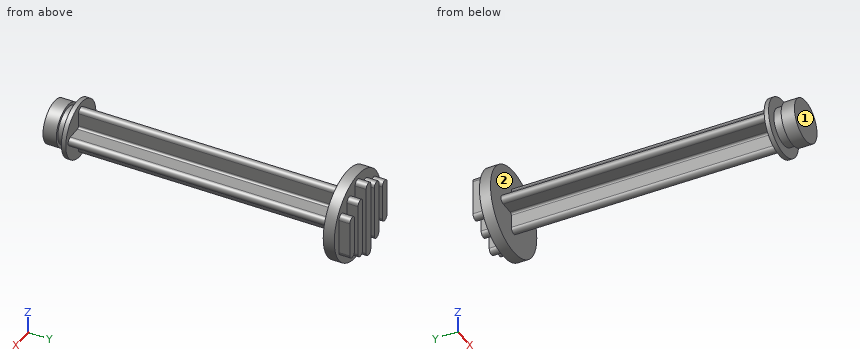
```python
from build123d import *

# Parameters (mm, degrees)
BOSS_EXTRUDE1_DEPTH = 60
SKETCH3_R           = 10
BOSS_EXTRUDE2_DEPTH = 2.5
BOSS_EXTRUDE3_DEPTH = 2.5


with BuildPart() as part:
    # Sketch1 → Revolve1 (revolve)
    with BuildSketch(Plane.XY):
        Polygon((0, 0), (4.875, 0), (4.875, 3), (4.225, 3), (4.225, 5), (6.5, 5), (6.5, 6), (0, 6), align=None)
    revolve(axis=Axis((0, 6, 0), (0, -1, 0)))

    # Sketch2 → Boss-Extrude1 (add)
    with BuildSketch(Plane(origin=(0, 6, 0), x_dir=(1, 0, 0), z_dir=(0, 1, 0))):
        with BuildLine():
            Line((-1, 4.5), (-1, 1.5))
            ThreePointArc((-1, 1.5), (-1.146446609, 1.146446609), (-1.5, 1))
            Line((-1.5, 1), (-4.5, 1))
            ThreePointArc((-4.5, 1), (-5.5, 0), (-4.5, -1))
            Line((-4.5, -1), (-1.5, -1))
            ThreePointArc((-1.5, -1), (-1.146446609, -1.146446609), (-1, -1.5))
            Line((-1, -1.5), (-1, -4.5))
            ThreePointArc((-1, -4.5), (0, -5.5), (1, -4.5))
            Line((1, -4.5), (1, -1.5))
            ThreePointArc((1, -1.5), (1.146446609, -1.146446609), (1.5, -1))
            Line((1.5, -1), (4.5, -1))
            ThreePointArc((4.5, -1), (5.5, 0), (4.5, 1))
            Line((4.5, 1), (1.5, 1))
            ThreePointArc((1.5, 1), (1.146446609, 1.146446609), (1, 1.5))
            Line((1, 1.5), (1, 4.5))
            ThreePointArc((1, 4.5), (0, 5.5), (-1, 4.5))
        make_face()
    extrude(amount=BOSS_EXTRUDE1_DEPTH)

    # Sketch3 → Boss-Extrude2 (add)
    with BuildSketch(Plane(origin=(0, 66, 0), x_dir=(1, 0, 0), z_dir=(0, 1, 0))):
        Circle(SKETCH3_R)
    extrude(amount=BOSS_EXTRUDE2_DEPTH)

    # Sketch4 → Boss-Extrude3 (add)
    with BuildSketch(Plane(origin=(0, 68.5, 0), x_dir=(1, 0, 0), z_dir=(0, 1, 0))):
        with BuildLine():
            ThreePointArc((1, 8), (0, 9), (-1, 8))
            Line((-1, 8), (-1, -8))
            ThreePointArc((-1, -8), (0, -9), (1, -8))
            Line((1, -8), (1, 8))
        make_face()
        with BuildLine():
            ThreePointArc((-2.5, 6), (-3.5, 7), (-4.5, 6))
            Line((-4.5, 6), (-4.5, -6))
            ThreePointArc((-4.5, -6), (-3.5, -7), (-2.5, -6))
            Line((-2.5, -6), (-2.5, 6))
        make_face()
        with BuildLine():
            ThreePointArc((4.5, 6), (3.5, 7), (2.5, 6))
            Line((2.5, 6), (2.5, -6))
            ThreePointArc((2.5, -6), (3.5, -7), (4.5, -6))
            Line((4.5, -6), (4.5, 6))
        make_face()
        with BuildLine():
            ThreePointArc((6, 4), (7, 5), (8, 4))
            Line((8, 4), (8, -4))
            ThreePointArc((8, -4), (7, -5), (6, -4))
            Line((6, -4), (6, 4))
        make_face()
        with BuildLine():
            Line((-6, -4), (-6, 4))
            ThreePointArc((-6, 4), (-7, 5), (-8, 4))
            Line((-8, 4), (-8, -4))
            ThreePointArc((-8, -4), (-7, -5), (-6, -4))
        make_face()
    extrude(amount=BOSS_EXTRUDE3_DEPTH)


solid = part.part
```
Build history of the part. All positions in model axes, mm. Face numbers are marked on the shaded views. Round coordinates to 2 decimals unless told otherwise and drop trailing zeros. Write each loop counter-clockwise with the first axis right and the second up, starting at its lowest first coordinate (ties: lowest second). Pieces come first, ordered by that corner, then holes. Notation, with made-up numbers: (13, -30) -> (57, -30) arc R17 cw to (57, -19) -> close; hole circle Ø3 at (84, -15). An arc over 180 degrees is marked (long way). Put each result on its own line as item: value.
Item 1: Wall check: probe 1 along Y at (x, z) = (3.5, -1.75); probe 2 along Y at (x, z) = (3.5, 3.5); probe 3 along Y at (x, z) = (6.25, -5). Give the ranges that are in metal, low to high. Write a range as from..to.
Here are the results:
probe 1: y = 0..6, 66..71
probe 2: y = 5..6, 66..71
probe 3: y = 66..68.5
Item 2: Flat gauge pins, fed straight in: P1, Ø12, axis at x = -6.5, z = -6, coming from the +Y side; P2, Ø0.9, axis at y = 42.5, z = 3.5, coming from the -X side; P3, Ø0.9, axis at y = 33.5, z = -2.5, coming from the +X side; P4, Ø0.8, axis at y = 69.5, z = 0, coming from the +X side. Where does each tip first touch, or does it go through?
Here are the results:
P1: stops at y = 71
P2: stops at x = -1
P3: stops at x = 1
P4: stops at x = 8
Item 3: Two-plate mould, pull along Y, no slides. Class the marked faces 1 and 2: pulls with the +Y half, pulls with the -Y half, needs draft (parallel to the pull), parting line crosses it, or undercut.
Here are the results:
face 1: pulls with the -Y half
face 2: undercut
Item 4: Slice it at A-A, the plane y = 30. Give the cut face in (x, z).
Here are the results:
outline: (-4.5, -1) -> (-1.5, -1) arc R0.5 cw to (-1, -1.5) -> (-1, -4.5) arc R1 ccw to (1, -4.5) -> (1, -1.5) arc R0.5 cw to (1.5, -1) -> (4.5, -1) arc R1 ccw to (4.5, 1) -> (1.5, 1) arc R0.5 cw to (1, 1.5) -> (1, 4.5) arc R1 ccw to (-1, 4.5) -> (-1, 1.5) arc R0.5 cw to (-1.5, 1) -> (-4.5, 1) arc R1 ccw to start
Item 5: Slice it at C-C, the plane x = -3.5. Give the cut face in (y, z).
Here are the results:
outline: (0, -3.39) -> (3, -3.39) -> (3, -2.37) -> (5, -2.37) -> (5, -5.48) -> (6, -5.48) -> (6, -1) -> (66, -1) -> (66, -9.37) -> (68.5, -9.37) -> (68.5, -7) -> (71, -7) -> (71, 7) -> (68.5, 7) -> (68.5, 9.37) -> (66, 9.37) -> (66, 1) -> (6, 1) -> (6, 5.48) -> (5, 5.48) -> (5, 2.37) -> (3, 2.37) -> (3, 3.39) -> (0, 3.39) -> close
Item 6: Slice it at B-B, the plane x = 0. Give the cut face in (y, z) (3 decimals).
Here are the results:
outline: (0, -4.875) -> (3, -4.875) -> (3, -4.225) -> (5, -4.225) -> (5, -6.5) -> (6, -6.5) -> (6, -5.5) -> (66, -5.5) -> (66, -10) -> (68.5, -10) -> (68.5, -9) -> (71, -9) -> (71, 9) -> (68.5, 9) -> (68.5, 10) -> (66, 10) -> (66, 5.5) -> (6, 5.5) -> (6, 6.5) -> (5, 6.5) -> (5, 4.225) -> (3, 4.225) -> (3, 4.875) -> (0, 4.875) -> close
